The model under review builds one solid part; all positions refer to its coordinate system, in mm. Give positions to 0.01 mm unless a question says otherwise; leave off trailing zeros. Loops run counter-clockwise (first coordinate to the right, second up) from the corner with the lowest first, then second, coordinate; pieces in that order, holes last. Notation, with made-up numbers: M -39,43.25 L -18,43.25 A29 ccw -18,77.25 Z; hole C 62.5,68 d3. An arc over 180 degrees is marked long. Put each result on its own line as item: value. Start each with the question number.
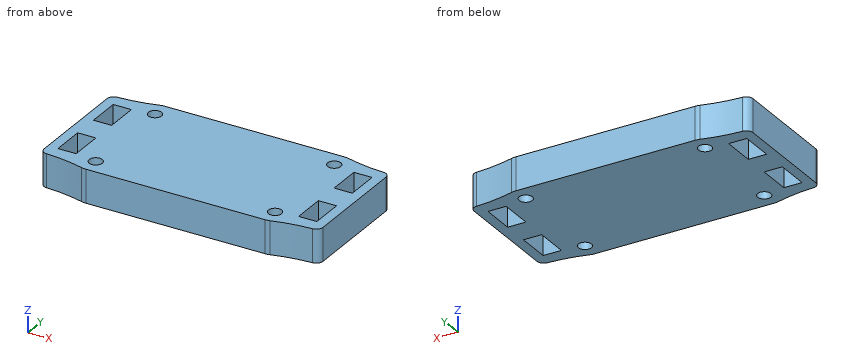
```python
from build123d import *

# Parameters (mm, degrees)
ESQUISSE1_R        = 1
ESQUISSE1_W        = 2.75
ESQUISSE1_H        = 5
BOSS_EXTRU_1_DEPTH = 5


with BuildPart() as part:
    # Esquisse1 → Boss.-Extru.1 (new body)
    with BuildSketch(Plane.XY):
        with BuildLine():
            Line((22.775862069, -16.426262466), (-4.224137931, -16.426262466))
            ThreePointArc((-4.224137931, -16.426262466), (-4.568324536, -16.402456235), (-4.905956113, -16.331490931))
            ThreePointArc((-4.905956113, -16.331490931), (-7.806629393, -15.692620747), (-10.762599469, -15.402273545))
            ThreePointArc((-10.762599469, -15.402273545), (-11.444714623, -15.096388709), (-11.724137931, -14.403013463))
            Line((-11.724137931, -14.403013463), (-11.724137931, 1.550488531))
            ThreePointArc((-11.724137931, 1.550488531), (-11.444714623, 2.243863776), (-10.762599469, 2.549748612))
            ThreePointArc((-10.762599469, 2.549748612), (-7.806629393, 2.840095814), (-4.905956113, 3.478965998))
            ThreePointArc((-4.905956113, 3.478965998), (-4.568324536, 3.549931303), (-4.224137931, 3.573737534))
            Line((-4.224137931, 3.573737534), (22.775862069, 3.573737534))
            ThreePointArc((22.775862069, 3.573737534), (23.120048674, 3.549931303), (23.457680251, 3.478965998))
            ThreePointArc((23.457680251, 3.478965998), (26.358353531, 2.840095814), (29.314323607, 2.549748612))
            ThreePointArc((29.314323607, 2.549748612), (29.996438761, 2.243863776), (30.275862069, 1.550488531))
            Line((30.275862069, 1.550488531), (30.275862069, -14.403013463))
            ThreePointArc((30.275862069, -14.403013463), (29.996438761, -15.096388709), (29.314323607, -15.402273545))
            ThreePointArc((29.314323607, -15.402273545), (26.358353531, -15.692620747), (23.457680251, -16.331490931))
            ThreePointArc((23.457680251, -16.331490931), (23.120048674, -16.402456235), (22.775862069, -16.426262466))
        make_face()
        with Locations((-4.224137931, 1.073737534)):
            Circle(ESQUISSE1_R, mode=Mode.SUBTRACT)
        with Locations((22.775862069, 1.073737534)):
            Circle(ESQUISSE1_R, mode=Mode.SUBTRACT)
        with Locations(Location((22.775862069, -13.926262466, 0), (0, 0, 180))):
            Circle(ESQUISSE1_R, mode=Mode.SUBTRACT)
        with Locations(Location((-4.224137931, -13.926262466, 0), (0, 0, 180))):
            Circle(ESQUISSE1_R, mode=Mode.SUBTRACT)
        with Locations((27.400862069, -10.926262466)):
            Rectangle(ESQUISSE1_W, ESQUISSE1_H, mode=Mode.SUBTRACT)
        with Locations((-8.849137931, -1.926262466)):
            Rectangle(ESQUISSE1_W, ESQUISSE1_H, mode=Mode.SUBTRACT)
        with Locations((-8.849137931, -10.926262466)):
            Rectangle(ESQUISSE1_W, ESQUISSE1_H, mode=Mode.SUBTRACT)
        with Locations((27.400862069, -1.926262466)):
            Rectangle(ESQUISSE1_W, ESQUISSE1_H, mode=Mode.SUBTRACT)
    extrude(amount=BOSS_EXTRU_1_DEPTH)


solid = part.part
```
Item 1: To check wall thickness, follow L1, parallel to X at y = -10, z = 2.35; L2, parallel to X at y = -14, z = 2.9; L3, parallel to Y at x = -9.5, z = 4.65. State the ranges of each line that lie inside material, in increasing order. Write a range as [from, to].
Item 2: Consider section B-B, the plane x = 27. Write out the cut boundary in (y, z).
Item 3: Consider section A-A, the plane y = -1.25. Write out the cut boundary in (x, z).
Item 4: Clearance check with flat-ended pins moving along their axes: pin 1 Ø1.2 at (x, y) = (22.78, -13.93) entering from -Z; pin 2 Ø3 at (x, z) = (28, 2) entering from -Y; pin 3 Ø1.4 at (x, z) = (27, 1.5) entering from +Y; pin 4 Ø0.8 at (x, z) = (-9, 3.5) entering from +Y. State where each tip first meets the part, or that it passes through.
Item 5: Consider section C-C, the plane z = 2.15. Give the number of separate pieces and of enclosed holes in the cut face, plus the area to 3 significant figures.
Report:
1. L1: [-11.72, -10.22], [-7.47, 26.03], [28.78, 30.28]
1. L2: [-11.72, -5.22], [-3.23, 21.78], [23.77, 30.28]
1. L3: [-15.48, -13.43], [-8.43, -4.43], [0.57, 2.63]
2. outline: M -15.6,0 L -13.43,0 L -13.43,5 L -15.6,5 Z; M -8.43,0 L -4.43,0 L -4.43,5 L -8.43,5 Z; M 0.57,0 L 2.75,0 L 2.75,5 L 0.57,5 Z
3. outline: M -11.72,0 L -10.22,0 L -10.22,5 L -11.72,5 Z; M -7.47,0 L 26.03,0 L 26.03,5 L -7.47,5 Z; M 28.78,0 L 30.28,0 L 30.28,5 L 28.78,5 Z
4. pin 1: through
4. pin 2: y = -15.67
4. pin 3: y = 2.85
4. pin 4: y = 2.73
5. separate pieces: 1
5. enclosed holes: 8
5. area: 752 mm²
